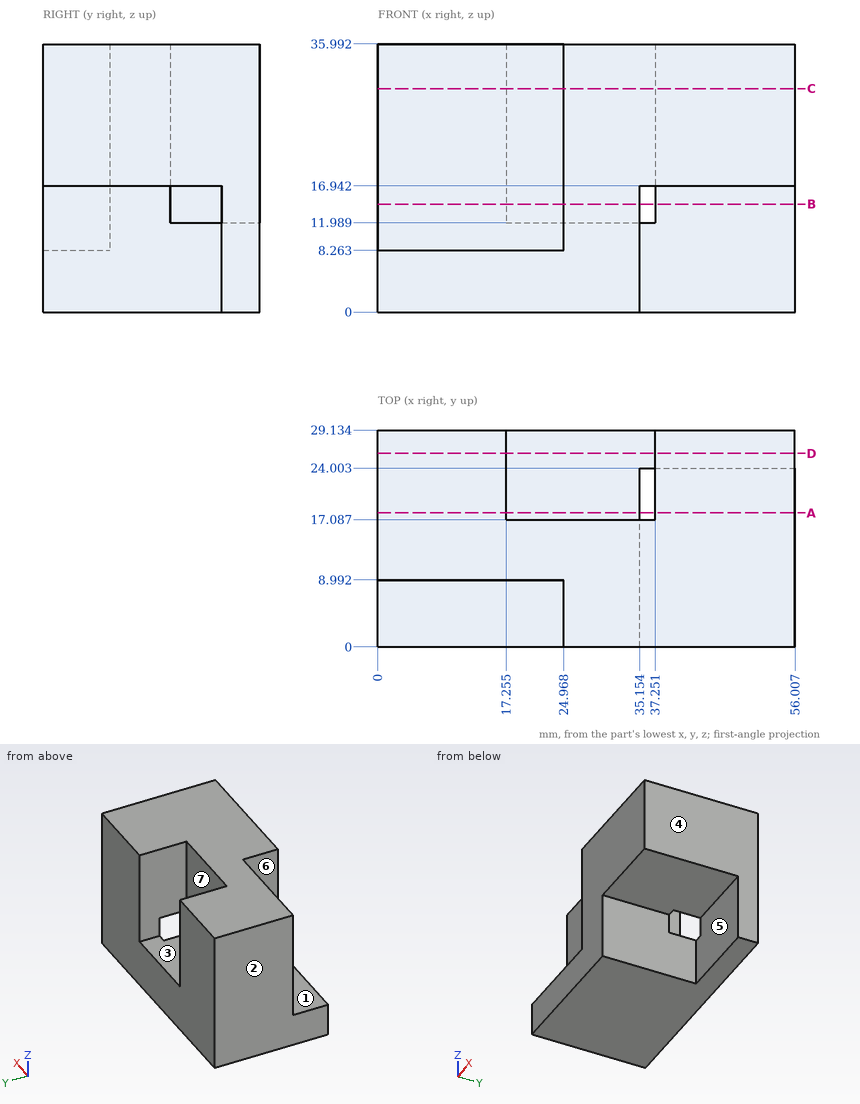
Source: three-view drawing plus pictorial views. Frame: mm from the lowest corner of the part. A direction names the side the tool comes from. Coordinates: 2 decimals unless noted, no trailing zeros. Loops run counter-clockwise (first coordinate to the right, second up) from the corner with the lowest first, then second, coordinate; pieces in that order, holes last. Notation, with made-up numbers: (86.5, 1) - (119.5, 1) arc R20 ccw to (119.5, 33) - close; hole circle Ø7 at (-24.5, 67). An arc over 180 degrees is marked (long way). One line per item, written item: value. Start each with the question number.
1. Section C-C (z = 30). Return the cut outline in (x, y) (1 decimal).
2. Section A-A (y = 18). Return the cut outline in (x, z) (1 decimal), and give its area (3 significant figures).
3. Section D-D (y = 26). Return the cut outline in (x, z) (1 decimal), and give its area (3 significant figures).
4. Ray query, L1, parallel to X at y = 23.75, z = 25.5 (1 decimal); L2, parallel to X at y = 5.75, z = 6; L3, parallel to Y at x = 34, z = 21.5. Return the intervals inside material, ascending.
5. Set-up query: the marked faces 5, 6 and 7. Return all of +Z, -Z, +X, -X, +Y, -Y with unobstructed straight access to the full face (end or side cutting, diameter ignored); none if empty.
6. Contact query for flat-ended pins moving along their axis: P1, Ø10, axis at x = 49, y = 11, coming from the -Z side; P2, Ø10, axis at x = 19, z = 27, coming from the -Y side; P3, Ø1, axis at y = 5, z = 32.5, coming from the -X side; P4, Ø1, axis at y = 26, z = 26, coming from the -X side. Output: stop coordinate, or through.
7. Mould query, pull axis X, two halves, no side actions, for the marked faces 1, 2, 3 and 4. Classes: pulls with the +X half, pulls with the -X half, needs draft (parallel to the pull), parting line crosses it, or undercut.
8. Section B-B (z = 14.5). Return the cut outline in (x, y) (1 decimal).
Verdict:
1. outline: (0, 9) - (25, 9) - (25, 0) - (56, 0) - (56, 29.1) - (37.3, 29.1) - (37.3, 17.1) - (17.3, 17.1) - (17.3, 29.1) - (0, 29.1) - close
2. outline: (0, 0) - (35.2, 0) - (35.2, 12) - (17.3, 12) - (17.3, 36) - (0, 36) - close; (37.3, 16.9) - (56, 16.9) - (56, 36) - (37.3, 36) - close
2. area: 1,190 mm2
3. outline: (0, 0) - (56, 0) - (56, 36) - (37.3, 36) - (37.3, 12) - (17.3, 12) - (17.3, 36) - (0, 36) - close
3. area: 1,540 mm2
4. L1: x = 0 to 17.3, 37.3 to 56
4. L2: x = 0 to 35.15
4. L3: y = 0 to 17.09
5. face 5: -Z, +X, -Y
5. face 6: +Z, -X, -Y
5. face 7: +Z, +Y
6. P1: stops at z = 16.94
6. P2: stops at y = 8.99
6. P3: stops at x = 24.97
6. P4: stops at x = 0
7. face 1: needs draft
7. face 2: pulls with the -X half
7. face 3: undercut
7. face 4: pulls with the +X half
8. outline: (0, 9) - (25, 9) - (25, 0) - (35.2, 0) - (35.2, 17.1) - (17.3, 17.1) - (17.3, 29.1) - (0, 29.1) - close; (37.3, 24) - (56, 24) - (56, 29.1) - (37.3, 29.1) - close
